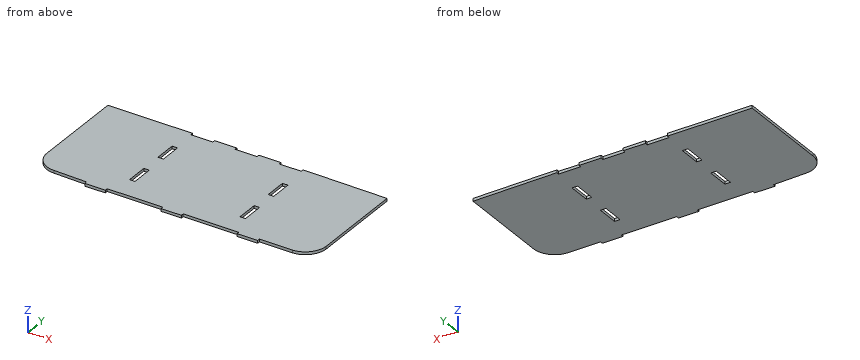
from build123d import *

# Parameters (mm, degrees)
SKETCH1_W           = 20.32
SKETCH1_H           = 81.316938585
SKETCH1_H_2         = 81.316938584
BOSS_EXTRUDE1_DEPTH = 10.16


with BuildPart() as part:
    # Sketch1 → Boss-Extrude1 (new body)
    # profile 1 of 2: a face of its own
    with BuildSketch(Plane.XY):
        with BuildLine():
            ThreePointArc((-520.699999986, 86.36), (-498.381536717, 32.478463279), (-444.5, 10.16))
            Line((-444.5, 10.16), (-321.2, 6.224098454))
            Line((-321.2, 6.224098454), (-321.2, -3.935901546))
            Line((-321.2, -3.935901546), (-245, -3.935901546))
            Line((-245, -3.935901546), (-245, 6.224098454))
            Line((-245, 6.224098454), (-38.1, 6.224098454))
            Line((-38.1, 6.224098454), (-38.1, -3.935901546))
            Line((-38.1, -3.935901546), (38.1, -3.935901546))
            Line((38.1, -3.935901546), (38.1, 6.224098454))
            Line((38.1, 6.224098454), (245, 6.224098454))
            Line((245, 6.224098454), (245, -3.935901546))
            Line((245, -3.935901546), (321.2, -3.935901546))
            Line((321.2, -3.935901546), (321.2, 6.224098454))
            Line((321.2, 6.224098454), (444.500003861, 6.224098454))
            add(Edge.make_bspline(
                [(444.500003861, 6.224098454), (516.375223264, 6.870661069), (520.046520409, 82.264098454)],
                knots=[3.150157412, 3.150157412, 3.150157412, 4.661289858, 4.661289858, 4.661289858], degree=2, weights=[1, 0.7278834, 1]))
            Line((520.046520409, 82.264098454), (520.070316171, 431.514078957))
            Line((520.070316171, 431.514078957), (205.706405146, 435.61))
            Line((205.706405146, 435.61), (205.558012439, 425.45))
            Line((205.558012439, 425.45), (123.444, 425.45))
            Line((123.444, 425.45), (123.444, 435.61))
            Line((123.444, 435.61), (41.148, 435.61))
            Line((41.148, 435.61), (41.148, 425.45))
            Line((41.148, 425.45), (-41.148, 425.45))
            Line((-41.148, 425.45), (-41.148, 435.61))
            Line((-41.148, 435.61), (-123.444, 435.61))
            Line((-123.444, 435.61), (-123.444, 425.45))
            Line((-123.444, 425.45), (-205.739999986, 425.45))
            Line((-205.739999986, 425.45), (-205.739999986, 388.35))
            Line((-205.739999986, 388.35), (-230.359692704, 388.35))
            Line((-230.359692704, 388.35), (-230.359692704, 435.61))
            Line((-230.359692704, 435.61), (-520.3601107, 435.61))
            Line((-520.3601107, 435.61), (-520.699999986, 86.36))
        make_face()
        with Locations((-206.375268781, 132.135407878)):
            Rectangle(SKETCH1_W, SKETCH1_H, mode=Mode.SUBTRACT)
        with Locations((206.375268781, 128.199506331)):
            Rectangle(SKETCH1_W, SKETCH1_H_2, mode=Mode.SUBTRACT)
        with Locations((-206.375268781, 294.769285048)):
            Rectangle(SKETCH1_W, SKETCH1_H, mode=Mode.SUBTRACT)
        with Locations((206.375268781, 290.833383501)):
            Rectangle(SKETCH1_W, SKETCH1_H, mode=Mode.SUBTRACT)
    # profile 2 of 2: a face of its own
    with BuildSketch(Plane.XY):
        Polygon((-205.739999986, 435.61), (-230.359692704, 435.61), (-230.359692704, 388.35), (-205.739999986, 388.35), (-205.739999986, 425.45), align=None)
    extrude(amount=BOSS_EXTRUDE1_DEPTH)


solid = part.part
Geometry: final body of the model. Coordinates: model frame, mm. Give positions to 0.01 mm unless a question says otherwise; leave off trailing zeros. Loops run counter-clockwise (first coordinate to the right, second up) from the corner with the lowest first, then second, coordinate; pieces in that order, holes last. Notation, with made-up numbers: M 17.5,18.5 L 22.5,18.5 A24 cw 22.5,52.5 Z; hole C -24.5,-7 d7. An arc over 180 degrees is marked long. Put each result on its own line as item: value. Start each with the question number.
1) Cut plane D-D (x = -18.5). Output: boundary loops of the cut face in (y, z).
2) Cut plane B-B (z = 4.75). Give the number of separate pieces and of enclosed holes in the cut face, then the cut area to 3 significant figures.
3) Cut plane C-C (x = 169). Output: boundary loops of the cut face in (y, z), then the cut area to 3 significant figures.
4) Ray query, line 1 along X through (y, z) = (292, 2.5); line 2 along X through (y, z) = (95, 6.25); line 3 along Y through (x, z) = (-38, 8.25). Return the intervals inside material, ascending.
5) Contact query for flat-ended pins moving along their axis: pin 1 (5 mm diameter, centred on y = 3, z = 5, fed in from -X); pin 2 (3 mm diameter, centred on x = -202, z = 4, fed in from +Y); pin 3 (5 mm diameter, centred on x = -167, z = 6, fed in from -Y). Output: stop coordinate, or through.
6) Cut plane A-A (y = 129). Output: boundary loops of the cut face in (x, z).
Verdict:
1. outline: M -3.94,0 L 425.45,0 L 425.45,10.16 L -3.94,10.16 Z
2. separate pieces: 1
2. enclosed holes: 4
2. area: 436,000 mm2
3. outline: M 6.22,0 L 425.45,0 L 425.45,10.16 L 6.22,10.16 Z
3. area: 4,260 mm2
4. line 1: -520.5 to -216.54, -196.22 to 196.22, 216.54 to 520.06
4. line 2: -520.69 to -216.54, -196.22 to 196.22, 216.54 to 520.05
4. line 3: -3.94 to 425.45
5. pin 1: x = -321.2
5. pin 2: y = 425.45
5. pin 3: y = 6.22
6. outline: M -520.66,0 L -216.54,0 L -216.54,10.16 L -520.66,10.16 Z; M -196.22,0 L 196.22,0 L 196.22,10.16 L -196.22,10.16 Z; M 216.54,0 L 520.05,0 L 520.05,10.16 L 216.54,10.16 Z
